Build history of the part. All positions in model axes, mm. Give positions to 0.01 mm unless a question says otherwise; leave off trailing zeros. Write each loop counter-clockwise with the first axis right and the second up, starting at its lowest first coordinate (ties: lowest second). Pieces come first, ordered by that corner, then holes. Notation, with made-up numbers: M 53,41.5 L 71,41.5 A28 ccw 71,70.5 Z; hole C 33,-18.75 d8. An arc over 180 degrees is marked long. Return JSON: item names as keys, results as strings. Group by question number.
Q1. Band-saw the part on C-C, the plane z = 58. Give the cut face in (x, y), then the cut area to 3 significant figures.
Q2. Band-saw the part on A-A, the plane y = 0. Give the cut face in (x, z), then the cut area to 3 significant figures.
Q3. Wall check: probe 1 along Y at (x, z) = (0, 33.5); probe 2 along Y at (x, z) = (-5, 59.5) (3 decimals). Give the ranges that are in metal, low to high.
Q4. Pull direction X, two halves, no side cores. Call faces 1 (the cylindrical face through (6.466, -2.681, 40.454)), 2 (the flat face through (4, -6, 80)), 3 (the cylindrical face through (-1.73, -7.81, 41.98)): +X half, -X half, draft (parallel to the pull), parting line (faces both ways), or undercut.
Q5. Flat gauge pins, fed straight in: pin 1 Ø5 at (x, z) = (-1.5, 67.5) entering from -Y; pin 2 Ø5 at (y, z) = (4.5, 45) entering from -X; pin 3 Ø4 at (x, z) = (4, 49.5) entering from -Y; pin 4 Ø3 at (x, y) = (0, 4) entering from +Z. Where does each tip first touch, or does it go through?
from build123d import *

# Parameters (mm, degrees)
SCHIZZO1_R                   = 9.75
SCHIZZO1_R_2                 = 7
ESTRUSIONE_ESTRUSIONE1_DEPTH = 5
SCHIZZO3_R                   = 8
SCHIZZO3_R_2                 = 7
ESTRUSIONE_ESTRUSIONE2_DEPTH = 75
SMUSSO1_SIZE                 = 2
SCHIZZO4_R                   = 9.75
SCHIZZO4_R_2                 = 9
TAGLIO_ESTRUSIONE1_DEPTH     = 10


with BuildPart() as part:
    # Schizzo1 → Estrusione-Estrusione1 (new body)
    with BuildSketch(Plane.XY):
        Circle(SCHIZZO1_R)
        Circle(SCHIZZO1_R_2, mode=Mode.SUBTRACT)
    extrude(amount=ESTRUSIONE_ESTRUSIONE1_DEPTH)

    # Schizzo3 → Estrusione-Estrusione2 (add)
    with BuildSketch(Plane.XY.offset(5)):
        Circle(SCHIZZO3_R)
        Circle(SCHIZZO3_R_2, mode=Mode.SUBTRACT)
    extrude(amount=ESTRUSIONE_ESTRUSIONE2_DEPTH)

    # Smusso1
    smusso1_edges = [part.edges().sort_by_distance(p)[0] for p in [
        (-7, 0, 0),
    ]]
    chamfer(smusso1_edges, length=SMUSSO1_SIZE)

    # Schizzo4 → Taglio-Estrusione1 (cut)
    with BuildSketch(Plane(origin=(0, 0, 0), x_dir=(-1, 0, 0), z_dir=(0, 0, -1))):
        Circle(SCHIZZO4_R)
        Circle(SCHIZZO4_R_2, mode=Mode.SUBTRACT)
    extrude(amount=-TAGLIO_ESTRUSIONE1_DEPTH, mode=Mode.SUBTRACT)


solid = part.part
From the geometry:
{
 "1": {"outline": "C 0,0 d16; hole C 0,0 d14", "area": "47.1 mm^2"},
 "2": {"outline": "M -9,0 L -7,2 L -7,80 L -8,80 L -8,5 L -9,5 Z; M 7,2 L 9,0 L 9,5 L 8,5 L 8,80 L 7,80 Z", "area": "166 mm^2"},
 "3": {"probe 1": "y = -8 to -7, 7 to 8", "probe 2": "y = -6.245 to -4.899, 4.899 to 6.245"},
 "4": {"face 1": "undercut", "face 2": "draft", "face 3": "parting line"},
 "5": {"pin 1": "stops at y = -8", "pin 2": "stops at x = -7.75", "pin 3": "stops at y = -7.75", "pin 4": "passes through"}
}
